The listing builds one solid part. Answer for the finished solid, in the listing's coordinates (mm). A direction names the side the tool comes from. Round coordinates to 2 decimals unless told otherwise and drop trailing zeros. Write each loop counter-clockwise with the first axis right and the second up, starting at its lowest first coordinate (ties: lowest second). Pieces come first, ordered by that corner, then holes. Notation, with made-up numbers: (-32, 40.25) - (-8, 40.25) arc R26 cw to (-8, 56.25) - close; hole circle Ø4 at (79, 70). An arc over 180 degrees is marked (long way). Return JSON: item names as keys, results as strings. Group by question number.
(1) Find the intervals of material crossed by line 1 along Z through (x, y) = (1, -17); line 2 along Z through (x, y) = (1.25, 15.5); line 3 along Y through (x, z) = (-2.5, 6.5), in increasing order. Write a range as [from, to].
(2) Determine the mould class of faces 3 (the flat face through (1, 0, 12.7)), 4 (the flat face through (2.84, 19.3, 6.26)), 5 (the conical face through (-3.872, -12.687, 6.027)) for opening direction X: +X half, -X half, draft (parallel to the pull), parting line (faces both ways), or undercut.
(3) Which of the six approach directions +Z, -Z, +X, -X, +Y, -Y give full straight-line access (tool end or side, diameter ignored) to faces 1 (the conical face through (6.68, 12.82, 6.15)), 2 (the flat face through (2.838, -16.295, 6.261))?
(4) Section C-C, the plane y = -21 is taken. Write down the section's boundary in (x, z), then the cut area to 3 significant figures.
(5) Each of these flat-tipped pins is pushed along its axis until it touches: pin 1 (4 mm diameter, centred on y = 15, z = 2.5, fed in from -X); pin 2 (4 mm diameter, centred on x = -2, y = 17.5, fed in from -Z). Where does it stop, or does it pass through?
(6) Section B-B, the plane y = 20 is taken. Write down the section's boundary in (x, z), then the cut area to 3 significant figures.
```python
from build123d import *

# Parameters (mm, degrees)
F0_W           = 12.7
F0_H           = 48.29048
F1_DEPTH       = 12.7
F2_SIZE2       = 12.69999
F2_SIZE        = 12.69999
F3_SIZE2       = 12.69999
F3_SIZE        = 12.69999
F6_D           = 3.81
F6_DEPTH       = 6.35
F6_TIP         = 1.1446394792
F6_ON_F4_D     = 3.81
F6_ON_F4_DEPTH = 6.35
F6_ON_F4_TIP   = 1.1446394792


# Not quite as in the source:
# - a fillet or chamfer is up to 0.001 mm smaller than in the source, because OpenCascade refuses the exact size


with BuildPart() as f1:
    # F0 (on Top) → F1 (new body)
    with BuildSketch(Plane.XY):
        with Locations((1.3377478731, 0)):
            Rectangle(F0_W, F0_H)
    extrude(amount=F1_DEPTH)

    # F2 (size 12.7 and 12.7 in the source; OpenCascade refuses exactly that, so slightly less here)
    f2_edges = [f1.edges().sort_by_distance(p)[0] for p in [
        (7.687748, -24.14524, 6.35),
    ]]
    chamfer(f2_edges, length=F2_SIZE, length2=F2_SIZE2)

    # F3 (size 12.7 and 12.7 in the source; OpenCascade refuses exactly that, so slightly less here)
    f3_edges = [f1.edges().sort_by_distance(p)[0] for p in [
        (-5.012252, 24.14524, 6.35),
    ]]
    chamfer(f3_edges, length=F3_SIZE, length2=F3_SIZE2)

    # F6
    with Locations(Plane(origin=(9.5664939365, -9.5664939365, 0), x_dir=(0.7071067812, 0.7071067812, 0), z_dir=(0.7071067812, -0.7071067812, 0))):
        with Locations((-11.6371181632, 6.35)):
            Hole(F6_D / 2, depth=F6_DEPTH)
            with Locations((0, 0, -(F6_DEPTH + F6_TIP / 2))):  # 118° drill point
                Cone(0, F6_D / 2, F6_TIP, mode=Mode.SUBTRACT)

    # F6 on F4
    with Locations(Plane(origin=(-8.2287460635, 8.2287460635, 0), x_dir=(-0.7071067812, -0.7071067812, 0), z_dir=(-0.7071067812, 0.7071067812, 0))):
        with Locations((-13.5289793484, 6.35)):
            Hole(F6_ON_F4_D / 2, depth=F6_ON_F4_DEPTH)
            with Locations((0, 0, -(F6_ON_F4_DEPTH + F6_ON_F4_TIP / 2))):  # 118° drill point
                Cone(0, F6_ON_F4_D / 2, F6_ON_F4_TIP, mode=Mode.SUBTRACT)


solid = f1.part
```
Working result:
{
 "1": {"line 1": "z = [0, 4.47], [8.23, 12.7]", "line 2": "z = [0, 5.46], [7.24, 12.7]", "line 3": "y = [-21.63, -16.64], [-12.14, 13.96]"},
 "2": {"face 3": "draft", "face 4": "-X half", "face 5": "undercut"},
 "3": {"face 1": "none", "face 2": "+Z, -Z, +X, -Y"},
 "4": {"outline": "(-5.01, 0) - (-1.87, 0) - (-1.87, 12.7) - (-5.01, 12.7) - close", "area": "39.9 mm^2"},
 "5": {"pin 1": "stops at x = -3.46", "pin 2": "passes through"},
 "6": {"outline": "(3.54, 0) - (7.69, 0) - (7.69, 12.7) - (3.54, 12.7) - close", "area": "52.6 mm^2"}
}
